Model file for the job. Use its own axes, mm. Coordinates: 2 decimals unless noted, no trailing zeros. Write each loop counter-clockwise with the first axis right and the second up, starting at its lowest first coordinate (ties: lowest second). Pieces come first, ordered by that corner, then holes. Notation, with made-up numbers: M 56,50 L 107,50 A19 cw 107,63 Z; hole C 50,14 d7. An arc over 180 degrees is marked long. Use CSV: the item, a comma, the result in double quotes. Start each with the question number.
from build123d import *

# Parameters (mm, degrees)
SKETCH_2_R      = 4
SKETCH_2_R_2    = 2
EXTRUDE_1_DEPTH = 6
CHAMFER_1_SIZE  = 0.2


with BuildPart() as part:
    # 草图2 → 凸台-拉伸1 (new, symmetric)
    with BuildSketch(Plane.XY):
        Circle(SKETCH_2_R)
        Circle(SKETCH_2_R_2, mode=Mode.SUBTRACT)
    extrude(amount=EXTRUDE_1_DEPTH, both=True)

    # 倒角1
    chamfer_1_edges = [part.edges().sort_by_distance(p)[0] for p in [
        (-4, 0, -6),
        (-4, 0, 6),
        (-2, 0, -6),
        (-2, 0, 6),
    ]]
    chamfer(chamfer_1_edges, length=CHAMFER_1_SIZE)


solid = part.part
1) Band-saw the part on C-C on z = 3. List the corners of the cut face in (x, y), then the cut area to 3 significant figures.
2) Band-saw the part on A-A on y = 0. List the corners of the cut face in (x, z).
3) Drop flat-ended pins along their axis: P1, Ø2, axis at y = -1.5, z = 2.5, coming from the +X side; P2, Ø2, axis at y = 2, z = -4, coming from the +X side; P3, Ø3, axis at x = 0, y = 0, coming from the -Z side. Give the stop position or say it passes through.
4) Wall check: L1, parallel to Y at x = 0, z = -1.75; L2, parallel to Y at x = -1.25, z = 4.5; L3, parallel to X at y = -1, z = -3.25. Give the ranges that are in metal, low to high. Write a range as [from, to].
5) Two-plate mould, pull along X, no slides. Class faces 1 (the face through (2, -2, 6)), 2 (the face through (-0.867, -3.905, 0.081)), 3 (the face through (0, -2, 0)): pulls with the +X half, pulls with the -X half, needs draft (parallel to the pull), parting line crosses it, or undercut.
Findings below:
1,outline,"C 0,0 d8; hole C 0,0 d4"
1,area,"37.7 mm2"
2,outline,"M -4,-5.8 L -3.8,-6 L -2.2,-6 L -2,-5.8 L -2,5.8 L -2.2,6 L -3.8,6 L -4,5.8 Z; M 2,-5.8 L 2.2,-6 L 3.8,-6 L 4,-5.8 L 4,5.8 L 3.8,6 L 2.2,6 L 2,5.8 Z"
3,P1,"stops at x = 3.97"
3,P2,"stops at x = 3.87"
3,P3,"passes through"
4,L1,"y = [-4, -2], [2, 4]"
4,L2,"y = [-3.8, -1.56], [1.56, 3.8]"
4,L3,"x = [-3.87, -1.73], [1.73, 3.87]"
5,face 1,"needs draft"
5,face 2,"parting line crosses it"
5,face 3,"undercut"
